Can you work these out from the drawing? Everything is in mm from the part's minimum corner. A direction names the side the tool comes from. Round coordinates to 2 decimals unless told otherwise and drop trailing zeros. Order: outer loops, then holes, each group sorted by start corner. A loop starts at its lowest first (then second) coordinate and runs counter-clockwise, first axis right, second up. Notation, with made-up numbers: (-18.5, 13) -> (22.5, 13) arc R25 ccw to (22.5, 33) -> close; hole circle Ø1 at (0.25, 74.5). An arc over 180 degrees is marked (long way). Use a Markdown table: item, result. Add a question column.
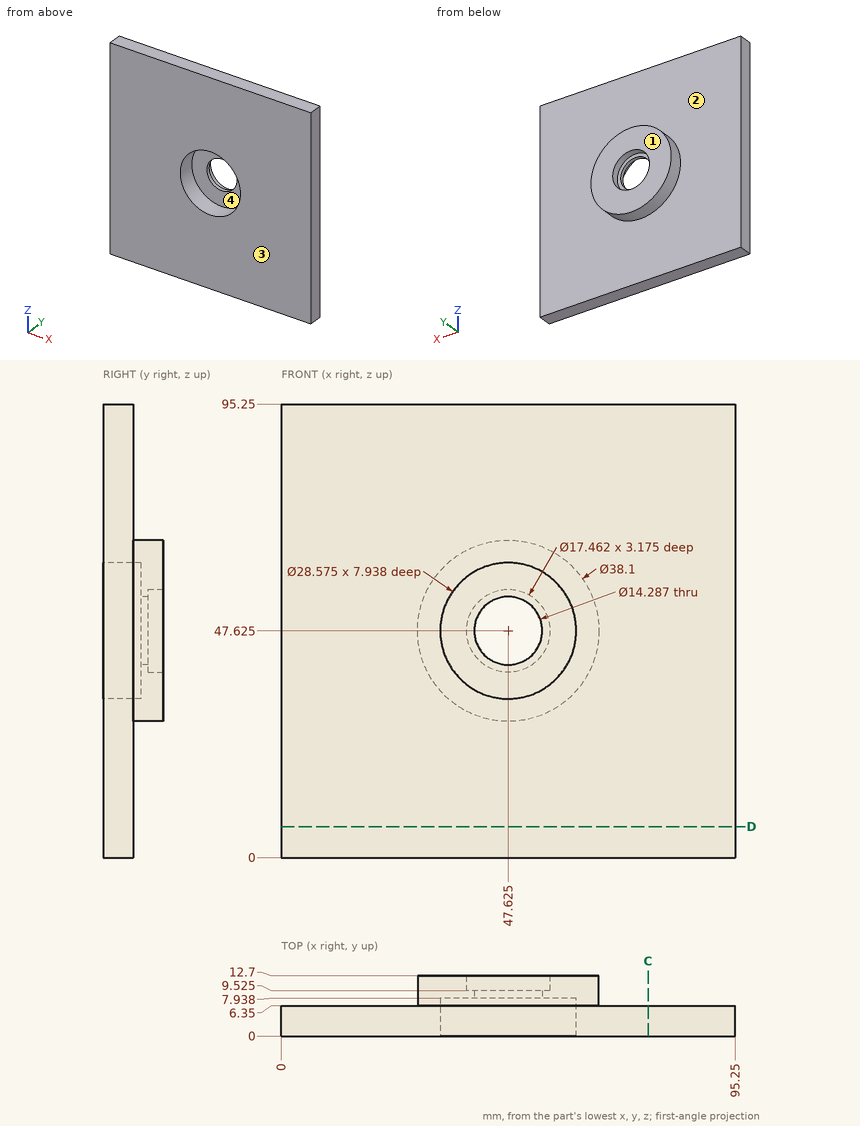
(1) On a 3-axis mill with a long thin cutter (end or side, diameter ignored), from which of +Z, -Z, +X, -X, +Y, -Y can I reach the whole of each face in a straight line? I mean the marked faces 1 and 2. Say none if no direction works.
(2) I want a section at D-D on z = 6.5. List the corners of the cut face in (x, y) for me, and give its area (3 significant figures).
(3) I'm going to push flat-ended pins straight in: P1, Ø8.5, axis at x = 54, z = 44.5, coming from the -Y side; P2, Ø2, axis at x = 58.5, y = 8, coming from the -Z side (1 decimal); P3, Ø1, axis at x = 36.5, y = 8, coming from the +Z side; P4, Ø13, axis at x = 47.625, z = 47.625, coming from the -Y side. Where does each tip first touch, or does it pass through?
(4) If we mould it in two halves opening along X, with no side actions, what happens to the marked faces 3 and 4? For each: pulls with the +X half, pulls with the -X half, needs draft (parallel to the pull), parting line crosses it, or undercut.
(5) I want a section at C-C on x = 77. List the corners of the cut face in (y, z) for me, and give its area (3 significant figures).
(6) Please list where these lines run through material, in increasing order: probe 1 along Z at (x, y) = (47.5, 11.75) (1 decimal); probe 2 along Y at (x, z) = (55.5, 20); probe 3 along X at (y, z) = (12.25, 53.5) (1 decimal). Write a range as from..to.
Output:
| question | item | result |
|---|---|---|
| 1 | face 1 | +Z, -Z, +X, -X, +Y |
| 1 | face 2 | +Y |
| 2 | outline | (0, 0) -> (95.25, 0) -> (95.25, 6.35) -> (0, 6.35) -> close |
| 2 | area | 605 mm² |
| 3 | P1 | y = 7.94 |
| 3 | P2 | z = 31.3 |
| 3 | P3 | z = 63.44 |
| 3 | P4 | through |
| 4 | face 3 | needs draft |
| 4 | face 4 | undercut |
| 5 | outline | (0, 0) -> (6.35, 0) -> (6.35, 95.25) -> (0, 95.25) -> close |
| 5 | area | 605 mm² |
| 6 | probe 1 | 28.6..38.9, 56.4..66.7 |
| 6 | probe 2 | 0..6.35 |
| 6 | probe 3 | 29.5..41.2, 54.1..65.7 |
